Build history of the part. All positions in model axes, mm. Round coordinates to 2 decimals unless told otherwise and drop trailing zeros. Write each loop counter-clockwise with the first axis right and the second up, starting at its lowest first coordinate (ties: lowest second). Pieces come first, ordered by that corner, then holes.
1) Saw through at A-A (y = -67.5). Write the cut outline in (x, z), plus the area to 3 significant figures.
2) Wall check: probe 1 along Y at (x, z) = (0, 0.9); probe 2 along Y at (x, z) = (-2, 0.65); probe 3 along X at (y, z) = (24, 0.1). Give the ranges that are in metal, low to high.
3) Flat gauge pin, fed straight in: pin 1 (2 mm diameter, centred on x = 1.5, y = -28.5, fed in from -Z). Where does the tip first touch, or does it go through?
4) Saw through at C-C (z = 1.2). Write the cut outline in (x, y).
5) Saw through at B-B (x = 0). Write the cut outline in (y, z), plus the area to 3 significant figures.
from build123d import *

# Parameters (mm, degrees)
SKETCH_1_W        = 45
SKETCH_1_H        = 180
EXTRUDE_1_DEPTH   = 2
CHAMFER_1_SIZE    = 2
HOLE_WIZARD_M81_D = 9


with BuildPart() as part:
    # Эскиз1 → Бобышка-Вытянуть1 (new body)
    with BuildSketch(Plane.XY):
        Rectangle(SKETCH_1_W, SKETCH_1_H)
    extrude(amount=EXTRUDE_1_DEPTH)

    # Фаска1
    chamfer_1_edges = [part.edges().sort_by_distance(p)[0] for p in [
        (22.5, -90, 1),
        (-22.5, -90, 1),
        (-22.5, 90, 1),
        (22.5, 90, 1),
    ]]
    chamfer(chamfer_1_edges, length=CHAMFER_1_SIZE)

    # Отверстие с зазором M81 (through all)
    with Locations(Plane.XY.offset(2)):
        with Locations((0, 67.5), (0, 22.5), (0, -22.5), (0, -67.5)):
            Hole(HOLE_WIZARD_M81_D / 2)


solid = part.part
Evaluation:
1. outline: (-22.5, 0) - (-4.5, 0) - (-4.5, 2) - (-22.5, 2) - close; (4.5, 0) - (22.5, 0) - (22.5, 2) - (4.5, 2) - close
1. area: 72.0 mm2
2. probe 1: y = -90 to -72, -63 to -27, -18 to 18, 27 to 63, 72 to 90
2. probe 2: y = -90 to -71.53, -63.47 to -26.53, -18.47 to 18.47, 26.53 to 63.47, 71.53 to 90
2. probe 3: x = -22.5 to -4.24, 4.24 to 22.5
3. pin 1: stops at z = 0
4. outline: (-22.5, -88) - (-20.5, -90) - (20.5, -90) - (22.5, -88) - (22.5, 88) - (20.5, 90) - (-20.5, 90) - (-22.5, 88) - close; hole circle Ø9 at (0, -67.5); hole circle Ø9 at (0, -22.5); hole circle Ø9 at (0, 22.5); hole circle Ø9 at (0, 67.5)
5. outline: (-90, 0) - (-72, 0) - (-72, 2) - (-90, 2) - close; (-63, 0) - (-27, 0) - (-27, 2) - (-63, 2) - close; (-18, 0) - (18, 0) - (18, 2) - (-18, 2) - close; (27, 0) - (63, 0) - (63, 2) - (27, 2) - close; (72, 0) - (90, 0) - (90, 2) - (72, 2) - close
5. area: 288 mm2
